from build123d import *

# Parameters (mm, degrees)
SKETCH_1_R             = 3
SKETCH_1_R_2           = 1.5
EXTRUDE_1_DEPTH        = 4
HOLE_WIZARD_M2_1_D     = 1.6
HOLE_WIZARD_M2_1_DEPTH = 14
HOLE_WIZARD_M2_1_TIP   = 0.480688495
CHAMFER_1_SIZE         = 2
CHAMFER_1_SIZE2        = 1.678199262
CHAMFER_1_PART_2_SIZE  = 2
CHAMFER_1_PART_2_SIZE2 = 1.678199262
CHAMFER_1_PART_3_SIZE  = 2
CHAMFER_1_PART_3_SIZE2 = 1.678199262
CHAMFER_1_PART_4_SIZE  = 2
CHAMFER_1_PART_4_SIZE2 = 1.678199262


with BuildPart() as part:
    # 草图1 → 凸台-拉伸1 (new body)
    with BuildSketch(Plane.XY):
        Polygon((0, 0), (44.599947574, 0), (49.869528236, -2.457245818), (52.827856068, 3.886908691), (48.296317133, 6), (32, 6), (32, 9), (28.867245682, 14.426089647), (23.980690184, 14.959516489), (20.872106338, 12.442234925), (21.220729309, 8.457456133), (19.5, 6), (3.635239529, 6), (-1.719029256, 9.749099364), (-5.73406431, 4.015035054), align=None)
        with Locations((26, 10)):
            Circle(SKETCH_1_R, mode=Mode.SUBTRACT)
        with Locations((-1.26909065, 5.1613379)):
            Circle(SKETCH_1_R_2, mode=Mode.SUBTRACT)
        with Locations((48.629768791, 1.982686222)):
            Circle(SKETCH_1_R_2, mode=Mode.SUBTRACT)
    extrude(amount=EXTRUDE_1_DEPTH)

    # M2 螺纹孔1
    with Locations(Plane.XY.offset(4)):
        with Locations((14, 2), (22, 2)):
            Hole(HOLE_WIZARD_M2_1_D / 2, depth=HOLE_WIZARD_M2_1_DEPTH)
            with Locations((0, 0, -(HOLE_WIZARD_M2_1_DEPTH + HOLE_WIZARD_M2_1_TIP / 2))):  # 118° drill point
                Cone(0, HOLE_WIZARD_M2_1_D / 2, HOLE_WIZARD_M2_1_TIP, mode=Mode.SUBTRACT)

    # 倒角1
    chamfer_1_edges = [part.edges().sort_by_distance(p)[0] for p in [
        (-5.73406431, 4.015035054, 2),
    ]]
    chamfer_1_side = [part.faces().sort_by_distance(p)[0] for p in [
        (-3.726546783, 6.882067209, 2),
    ]]
    chamfer(chamfer_1_edges, length=CHAMFER_1_SIZE, length2=CHAMFER_1_SIZE2, reference=chamfer_1_side[0])

    # 倒角1 part 2
    chamfer_1_part_2_edges = [part.edges().sort_by_distance(p)[0] for p in [
        (-1.719029256, 9.749099364, 2),
    ]]
    chamfer_1_part_2_side = [part.faces().sort_by_distance(p)[0] for p in [
        (0.958105137, 7.874549682, 2),
    ]]
    chamfer(chamfer_1_part_2_edges, length=CHAMFER_1_PART_2_SIZE, length2=CHAMFER_1_PART_2_SIZE2, reference=chamfer_1_part_2_side[0])

    # 倒角1 part 3
    chamfer_1_part_3_edges = [part.edges().sort_by_distance(p)[0] for p in [
        (52.827856068, 3.886908691, 2),
    ]]
    chamfer_1_part_3_side = [part.faces().sort_by_distance(p)[0] for p in [
        (51.348692152, 0.714831437, 2),
    ]]
    chamfer(chamfer_1_part_3_edges, length=CHAMFER_1_PART_3_SIZE, length2=CHAMFER_1_PART_3_SIZE2, reference=chamfer_1_part_3_side[0])

    # 倒角1 part 4
    chamfer_1_part_4_edges = [part.edges().sort_by_distance(p)[0] for p in [
        (49.869528236, -2.457245818, 2),
    ]]
    chamfer_1_part_4_side = [part.faces().sort_by_distance(p)[0] for p in [
        (47.234737905, -1.228622909, 2),
    ]]
    chamfer(chamfer_1_part_4_edges, length=CHAMFER_1_PART_4_SIZE, length2=CHAMFER_1_PART_4_SIZE2, reference=chamfer_1_part_4_side[0])


solid = part.part
The listing builds one solid part. Answer for the finished solid, in the listing's coordinates (mm). A direction names the side the tool comes from. Give positions to 0.01 mm unless a question says otherwise; leave off trailing zeros. Loops run counter-clockwise (first coordinate to the right, second up) from the corner with the lowest first, then second, coordinate; pieces in that order, holes last. Notation, with made-up numbers: (12.5, 79) - (49.5, 79) arc R22 ccw to (49.5, 88) - close; hole circle Ø10 at (10, 32). An arc over 180 degrees is marked (long way). Write each question's results on one line, items separated by ' | '.
1. Find section A-A, the plane x = 27.5. Write down the section's boundary in (y, z).
Resolved:
outline: (0, 0) - (7.4, 0) - (7.4, 4) - (0, 4) - close; (12.6, 0) - (14.58, 0) - (14.58, 4) - (12.6, 4) - close
2. Flat-ended cylindrical pins translate along their axes: P1, Ø1.2, axis at x = 12.5, z = 2, coming from the -Y side; P2, Ø0.9, axis at y = 7.5, z = 3, coming from the +X side; P3, Ø1.2, axis at x = 15, z = 3, coming from the +Y side. Find the tip coordinate at first contact, or state that the pin passes through.
Resolved:
P1: stops at y = 0 | P2: stops at x = 32 | P3: stops at y = 6
3. Which of the six approach directions +Z, -Z, +X, -X, +Y, -Y give full straight-line access (tool end or side, diameter ignored) to faces 4 (the face through (22, 0, 2)), 5 (the face through (1.803, 7.283, 1.972)), 6 (the face through (14.63, 1.51, 1.97))?
Resolved:
face 4: +Z, -Z, -X, -Y | face 5: +Z, -Z, +Y | face 6: +Z, -Z
4. For a pull along X with two mould halves and no side action, classify faces 1 (the face through (21.63, 1.29, 1.97)), 2 (the face through (26.46, 14.69, 1.97)), 3 (the face through (-4.47, 4.33, 1.97)) as +X half, -X half, draft (parallel to the pull), parting line (faces both ways), or undercut.
Resolved:
face 1: undercut | face 2: +X half | face 3: -X half
5. Find section B-B, the plane y = 10. Write down the section's boundary in (x, z).
Resolved:
outline: (21.09, 0) - (23, 0) - (23, 4) - (21.09, 4) - close; (29, 0) - (31.42, 0) - (31.42, 4) - (29, 4) - close
6. Consider probe 1 along Y at (x, z) = (14, 0.3); probe 2 along X at (y, z) = (7.5, 1.75); probe 3 along X at (y, z) = (2.25, 1.4). Determine where each line is inside the solid, lowest interval first. Write a range as from..to.
Resolved:
probe 1: y = 0..1.2, 2.8..6 | probe 2: x = -3.29..1.49, 20.55..24.34, 27.66..32 | probe 3: x = -3.21..13.24, 14.76..21.24, 22.76..47.15, 50.11..51.94
7. Find section C-C, the plane z = 2.05. Write down the section's boundary in (x, y), then the cut area to 3 significant figures.
Resolved:
outline: (-4.59, 5.65) - (-4.36, 3.05) - (0, 0) - (44.6, 0) - (48.06, -1.61) - (50.58, -0.94) - (51.98, 2.07) - (51.31, 4.6) - (48.3, 6) - (32, 6) - (32, 9) - (28.87, 14.43) - (23.98, 14.96) - (20.87, 12.44) - (21.22, 8.46) - (19.5, 6) - (3.64, 6) - (-0.08, 8.6) - (-2.68, 8.37) - close; hole circle Ø3 at (-1.27, 5.16); hole circle Ø1.6 at (14, 2); hole circle Ø1.6 at (22, 2); hole circle Ø6 at (26, 10); hole circle Ø3 at (48.63, 1.98) | area: 385 mm^2
8. Find section D-D, the plane x = 40. Write down the section's boundary in (y, z).
Resolved:
outline: (0, 0) - (6, 0) - (6, 4) - (0, 4) - close
